Autodesk Inventor part; units mm, degrees
ref_plane "YZ Plane" through (0, 0, 0) normal (1, 0, 0) x (0, 1, 0)
ref_plane "XZ Plane" through (0, 0, 0) normal (0, 1, 0) x (-1, 0, 0)
ref_plane "XY Plane" through (0, 0, 0) normal (0, 0, 1) x (1, 0, 0)
sketch "スケッチ1" plane through (0, 0, 0) normal (0, 0, 1) x (1, 0, 0)
  circle A0 centre (0, 0) radius 33.5 construction
  circle A1 centre (0, 0) radius 43.5
  dimension "d0" = 67
  dimension "d1" = 87
extrude "押し出し1" add sketch "スケッチ1" along normal blind 1
sketch "スケッチ2" plane through (0, 0, 1) normal (0, 0, 1) x (1, 0, 0)
  circle A0 centre (0, 0) radius 33.5
  circle A1 centre (0, 0) radius 43.5
  dimension "d4" = 67
extrude "押し出し2" add sketch "スケッチ2" along normal blind 2
sketch "スケッチ4" plane through (0, 0, 3) normal (0, 0, 1) x (1, 0, 0)
  circle A0 centre (0, 0) radius 33.5 construction
  circle A1 centre (0, 0) radius 43.5 construction
  line L0 (0, 0) -> (33.5, 0) construction
  line L1 (33.5, 0) -> (43.5, 0) construction
  circle A2 centre (0, 0) radius 33.5 construction
  line L2 (0, 0) -> (-33.5, 0) construction
  circle A3 centre (0, 0) radius 43.5 construction
  line L3 (-43.5, 0) -> (-33.5, 0) construction
  circle A4 centre (38.5, 0) radius 3.05
  circle A5 centre (-38.5, 0) radius 3.05
  circle A6 centre (0, 0) radius 38.5 construction
  circle A7 centre (-9.9645, 37.1881) radius 3.05 construction
  arc A8 (-3.4944, 44.3648) -> (-9.9645, 37.1881) centre (38.5, 0) ccw construction
  line L4 (38.5, 0) -> (-9.9645, 37.1881) construction
  line L5 (-9.9645, 37.1881) -> (-12.3843, 39.0449) construction
  arc A9 (0.0788, 43.4999) -> (-7.5448, 35.3314) centre (38.5, 0) ccw
  arc A10 (-9.6001, 42.4274) -> (-12.3843, 39.0449) centre (38.5, 0) ccw
  arc A11 (-12.3843, 39.0449) -> (-7.5448, 35.3314) centre (-9.9645, 37.1881) ccw
  arc A12 (0.0788, 43.4999) -> (-9.6001, 42.4274) centre (0, 0) ccw
  circle A13 centre (9.9645, -37.1881) radius 3.05 construction
  line L6 (-38.5, 0) -> (9.9645, -37.1881) construction
  line L7 (9.9645, -37.1881) -> (12.3843, -39.0449) construction
  arc A14 (-0.0788, -43.4999) -> (7.5448, -35.3314) centre (-38.5, 0) ccw
  arc A15 (9.6001, -42.4274) -> (12.3843, -39.0449) centre (-38.5, 0) ccw
  arc A16 (12.3843, -39.0449) -> (7.5448, -35.3314) centre (9.9645, -37.1881) ccw
  arc A17 (-0.0788, -43.4999) -> (9.6001, -42.4274) centre (0, 0) ccw
  line L8 (-9.9645, 37.1881) -> (9.9645, -37.1881) construction
  dimension "d7" = 6.1
  dimension "d8" = 3.05
  dimension "d15" = 105
extrude "押し出し3" cut sketch "スケッチ4" against normal through all
fillet "フィレット1" radius 1 4 edges at (-9.6001, 42.4274, 1.5) (0.0788, 43.4999, 1.5) (-0.0788, -43.4999, 1.5) (9.6001, -42.4274, 1.5)
sketch "スケッチ6" plane through (0, 0, 3) normal (0, 0, 1) x (1, 0, 0)
  arc A0 (-12.3843, 39.0449) -> (-7.5448, 35.3314) centre (-9.9645, 37.1881) ccw construction
  circle A1 centre (38.5, 0) radius 3.05 construction
  circle A2 centre (-9.9645, 37.1881) radius 3
  circle A3 centre (38.5, 0) radius 3
  point P0 (0, 0)
  dimension "d16" = 6
extrude "押し出し5" add sketch "スケッチ6" along normal blind 0.1
sketch "スケッチ7" plane through (-9.9645, 37.1881, 3.1) normal (0, 0, 1) x (1, 0, 0)
  circle A0 centre (0, 0) radius 3 construction
  circle A1 centre (48.4645, -37.1881) radius 3 construction
  circle A2 centre (0, 0) radius 5
  circle A3 centre (48.4645, -37.1881) radius 3
  circle A4 centre (48.4645, -37.1881) radius 5
  point P0 (9.9645, -37.1881)
  dimension "d19" = 10
extrude "押し出し6" add sketch "スケッチ7" along normal blind 0.4 contours A2 | A3 | A4
sketch "スケッチ8" plane through (-9.9645, 37.1881, 3.5) normal (0, 0, 1) x (1, 0, 0)
  circle A0 centre (9.9645, -37.1881) radius 33.5 construction
  circle A1 centre (9.9645, -37.1881) radius 29 construction
  circle A2 centre (48.4645, -37.1881) radius 5 construction
  arc A3 (43.6349, -38.4822) -> (36.1372, -24.6985) centre (11.2764, -47.1527) ccw construction
  line L0 (9.9645, -37.1881) -> (48.4645, -37.1881) construction
  line L1 (48.4645, -37.1881) -> (11.2764, -47.1527) construction
  circle A4 centre (0, 0) radius 5 construction
  circle A5 centre (48.4645, -37.1881) radius 3.05 construction
  line L2 (48.4645, -37.1881) -> (-9.5202, 7.3051) construction
  line L3 (9.9645, -37.1881) -> (-4.6207, -1.9104) construction
  circle A6 centre (0, 0) radius 5 construction
  line L4 (-1.1156, -10.3883) -> (-7.9245, 6.0806)
  arc A7 (36.1372, -24.6985) -> (-1.1156, -10.3883) centre (9.9645, -37.1881) ccw
  arc A8 (43.6349, -38.4822) -> (36.1372, -24.6985) centre (11.2764, -47.1527) ccw
  arc A9 (22.6521, -78.7967) -> (10.4317, 6.3093) centre (9.9645, -37.1881) ccw
  arc A10 (43.6349, -38.4822) -> (53.4645, -37.1881) centre (48.4645, -37.1881) ccw
  arc A11 (53.4645, -37.1881) -> (5.2496, 6.0556) centre (9.9645, -37.1881) ccw
  line L5 (-7.9245, 6.0806) -> (-9.5202, 7.3051)
  line L6 (-9.5202, 7.3051) -> (-4.6501, 13.652)
  line L7 (-4.6501, 13.652) -> (5.2496, 6.0556)
  point P0 (10.4317, 6.3093)
  dimension "d22" = 58
  dimension "d23" = 15
  dimension "d24" = 12
  dimension "d25" = 8
extrude "押し出し7" add sketch "スケッチ8" along normal blind 2.5
sketch "スケッチ9" plane through (0, 0, 3) normal (0, 0, 1) x (1, 0, 0)
  circle A0 centre (0, 0) radius 61.8319
extrude "押し出し8" cut sketch "スケッチ9" against normal through all
sketch "スケッチ10" plane through (-9.9645, 37.1881, 3) normal (0, 0, -1) x (-1, 0, 0)
  circle A0 centre (-48.4645, -37.1881) radius 3 construction
  circle A1 centre (0, 0) radius 3 construction
  circle A2 centre (-48.4645, -37.1881) radius 1.3
  circle A3 centre (0, 0) radius 1.3
  point P0 (-9.9645, -37.1881)
  dimension "d30" = 2.6
extrude "押し出し9" cut sketch "スケッチ10" against normal through all
fillet "フィレット2" radius 3 6 edges at (-19.4848, 44.4933, 4.75) (-14.6147, 50.8401, 4.75) (-17.889, 43.2688, 4.75) (-4.7149, 43.2437, 4.75) (-11.0801, 26.7998, 4.75) (26.1727, 12.4896, 4.75)
sketch "スケッチ11" plane through (38.5, 0, 3) normal (0, 0, -1) x (-1, 0, 0)
  circle A0 centre (0, 0) radius 3
  circle A1 centre (0, 0) radius 5
  circle A2 centre (48.4645, 37.1881) radius 3
  circle A3 centre (48.4645, 37.1881) radius 5
  point P0 (38.5, 0)
extrude "押し出し10" add sketch "スケッチ11" against normal up to surface (0.1 mm away)
sketch "スケッチ12" plane through (-9.9645, 37.1881, 3.5) normal (0, 0, -1) x (-1, 0, 0)
  arc A0 (7.9351, 5.9159) -> (7.8609, 9.4676) centre (5.4809, 7.6413) ccw
  line L0 (6.4764, 11.2719) -> (7.8609, 9.4676)
  arc A1 (6.4764, 11.2719) -> (2.2701, 11.8257) centre (4.0964, 9.4456) ccw
  line L1 (-4.3131, 6.7742) -> (2.2701, 11.8257)
  arc A2 (-6.3862, 6.1644) -> (-4.3131, 6.7742) centre (-6.1394, 9.1543) ccw
  arc A3 (-6.3862, 6.1644) -> (-53.4645, -37.1881) centre (-9.9645, -37.1881) ccw
  arc A4 (-43.6349, -38.4822) -> (-53.4645, -37.1881) centre (-48.4645, -37.1881) ccw
  arc A5 (-36.4032, -24.9966) -> (-43.6349, -38.4822) centre (-11.2764, -47.1527) ccw
  arc A6 (-36.4032, -24.9966) -> (-35.9638, -24.3414) centre (-38.6534, -23.0124) ccw
  arc A7 (-1.4457, -9.4676) -> (-35.9638, -24.3414) centre (-9.9645, -37.1881) ccw
  arc A8 (-1.4457, -9.4676) -> (2.2079, -7.7461) centre (-0.5645, -6.5999) ccw
  line L2 (4.6207, -1.9104) -> (2.2079, -7.7461)
  circle A9 centre (0, 0) radius 5
  line L3 (7.6169, 5.3368) -> (4.6207, -1.9104)
  arc A10 (7.9351, 5.9159) -> (7.6169, 5.3368) centre (10.3893, 4.1906) ccw
extrude "押し出し11" add sketch "スケッチ12" along normal up to surface (0.5 mm away)
ref_plane "作業平面1" through (-8.5188, 27.7206, 3.5) normal (-0.5666562, -0.8239543, 0) x (0, 0, -1)
properties part number "canere_02_t3_01"
Can you work these out from the model? Positions are in its coordinate system, mm. A direction names the side the tool comes from. Coordinates: 2 decimals unless noted, no trailing zeros. Loops run counter-clockwise (first coordinate to the right, second up) from the corner with the lowest first, then second, coordinate; pieces in that order, holes last. Notation, with made-up numbers: (34.5, 31.5) -> (42.5, 31.5) arc R22 cw to (42.5, 49.5) -> close; hole circle Ø10 at (66, -3). An arc over 180 degrees is marked (long way). Put each result on its own line as item: value. Start each with the question number.
Q1. I want a section at A-A (x = 38.5). Write out the boundary of the cut face in (y, z), plus the area to 3 significant figures.
Q2. Thinking about a two-plate mould opening in X: for faces 3 (the face through (30.784, 5.962, 4.732)), 4 (the face through (39.252, -4.943, 3.246)), 5 (the face through (-10.71, 27.89, 4.77)), which applies, pulls with the +X half, pulls with the -X half, needs draft (parallel to the pull), parting line crosses it, or undercut?
Q3. I want a section at B-B (y = 41). Write out the boundary of the cut face in (x, z).
Q4. If I drill on line 1 (Y direction, x = -9.5, z = 3.9); line 2 (Y direction, x = 38.5, z = 3.8); line 3 (Y direction, x = -2, z = 5.8), over which ranges is the centre line in solid material (lowest first)? Write a range as [from, to].
Q5. I'm going to push flat-ended pins straight in: P1, Ø2.5, axis at x = 38.5, y = 0, coming from the -Z side; P2, Ø1.5, axis at x = -11, z = 5.5, coming from the -Y side. Where does each tip first touch, or does it pass through?
Q6. For faces 1 (the face through (39.252, -4.943, 4.732)), 2 (the face through (-1.59, 43.47, 4.73)), which set-ups out of +Z, -Z, +X, -X, +Y, -Y let a thin tool reach every point of the face, with its end or its side?
Q7. I want a section at C-C (x = 18.5). Write out the boundary of the cut face in (y, z).
Taken from the geometry:
1. outline: (-5, 3) -> (-1.3, 3) -> (-1.3, 6) -> (-5, 6) -> close; (1.3, 3) -> (20.25, 3) -> (20.25, 6) -> (1.3, 6) -> close
1. area: 67.9 mm2
2. face 3: pulls with the -X half
2. face 4: parting line crosses it
2. face 5: undercut
3. outline: (-16.95, 3) -> (14.53, 3) -> (14.53, 6) -> (-16.95, 6) -> close
4. line 1: y = [27.59, 35.97], [38.4, 46.92]
4. line 2: y = [-5, -1.3], [1.3, 20.25]
4. line 3: y = [28.93, 43.45]
5. P1: passes through
5. P2: stops at y = 27.71
6. face 1: +Z, -Z, -Y
6. face 2: +Z, -Z, +Y
7. outline: (22.33, 3) -> (39.37, 3) -> (39.37, 6) -> (22.33, 6) -> close
